Work out the finished part from the listing and answer in its coordinate system (mm). A direction names the side the tool comes from. Round coordinates to 2 decimals unless told otherwise and drop trailing zeros. Write each loop counter-clockwise with the first axis right and the second up, starting at its lowest first coordinate (ties: lowest second). Pieces come first, ordered by that corner, then holes.
1. A tool of negligible diameter and unlimited length cuts with its end or side. For faces 1 (the face through (103.216, 2.549, -5.514)), 2 (the face through (73.4, 1.6, -0.2)), 3 (the face through (15.24, 1.57, -18.86)), from which of +Z, -Z, +X, -X, +Y, -Y can it reach the whole face along a straight path? Write none if from no direction.
2. Find section B-B (y = 1.2). Count the separate pieces of the cut face and the enclosed holes in it, and give its area (3 significant figures).
3. Straight lines are drawn through the part: probe 1 along X at (y, z) = (0.65, -9.5); probe 2 along Z at (x, y) = (6.35, 1.8); probe 3 along X at (y, z) = (1.2, -10). For each, find the intervals that lie inside material, in ascending order.
4. Determine the mould class of faces 4 (the face through (56, 3.175, -10)), 5 (the face through (82.204, 2.549, -13.536)), 6 (the face through (0, 2, -10)) for opening direction X: pulls with the +X half, pulls with the -X half, needs draft (parallel to the pull), parting line crosses it, or undercut.
5. Find section C-C (x = 28). Write down the section's boundary in (y, z) (3 decimals), and give its area (3 significant figures).
6. Flat-ended cylindrical pins translate along their axes: pin 1 Ø2.5 at (x, z) = (92.71, -9.525) entering from -Y; pin 2 Ø6.5 at (x, z) = (88, -11) entering from +Y (3 decimals); pin 3 Ø1 at (y, z) = (1.5, -16) entering from +X; pin 4 Ø1.5 at (y, z) = (0.5, -3) entering from -X. Find the tip coordinate at first contact, or state that the pin passes through.
```python
from build123d import *

# Parameters (mm, degrees)
BOSS_EXTRUDE1_DEPTH          = 3.175
CUT_EXTRUDE2_DEPTH           = 1.27
F_1_8_0_125_DIAMETER_HOLE1_D = 3.175
CUT_EXTRUDE3_DEPTH           = 116.920115273
FILLET1_R                    = 15
F_1_8_0_125_DIAMETER_HOLE2_D = 3.175


with BuildPart() as part:
    # Sketch1 → Boss-Extrude1 (new body)
    with BuildSketch(Plane(origin=(0, 0, 0), x_dir=(1, 0, 0), z_dir=(0, 1, 0))):
        with BuildLine():
            Line((6.35, 0), (107.95, 0))
            ThreePointArc((107.95, 0), (112.440128061, 1.859871939), (114.3, 6.35))
            Line((114.3, 6.35), (114.3, 12.7))
            ThreePointArc((114.3, 12.7), (112.440128061, 17.190128061), (107.95, 19.05))
            Line((107.95, 19.05), (6.35, 19.05))
            ThreePointArc((6.35, 19.05), (1.859871939, 17.190128061), (0, 12.7))
            Line((0, 12.7), (0, 6.35))
            ThreePointArc((0, 6.35), (1.859871939, 1.859871939), (6.35, 0))
        make_face()
    extrude(amount=BOSS_EXTRUDE1_DEPTH)

    # Sketch4 → Cut-Extrude2 (cut)
    with BuildSketch(Plane(origin=(0, 3.175, 0), x_dir=(1, 0, 0), z_dir=(0, 1, 0))):
        with BuildLine():
            Line((109.744274308, 12.384881715), (96.868569632, 14.655215845))
            ThreePointArc((96.868569632, 14.655215845), (92.71, 16.129), (88.551430368, 14.655215845))
            Line((88.551430368, 14.655215845), (75.675725692, 12.384881715))
            ThreePointArc((75.675725692, 12.384881715), (73.276, 9.525), (75.675725692, 6.665118285))
            Line((75.675725692, 6.665118285), (88.551430368, 4.394784155))
            ThreePointArc((88.551430368, 4.394784155), (92.71, 2.921), (96.868569632, 4.394784155))
            Line((96.868569632, 4.394784155), (109.744274308, 6.665118285))
            ThreePointArc((109.744274308, 6.665118285), (112.144, 9.525), (109.744274308, 12.384881715))
        make_face()
    extrude(amount=-CUT_EXTRUDE2_DEPTH, mode=Mode.SUBTRACT)

    # 1/8 (0.125) Diameter Hole1 (through all)
    with Locations(Plane(origin=(0, 3.175, 0), x_dir=(1, 0, 0), z_dir=(0, 1, 0))):
        with Locations((6.35, 9.525)):
            Hole(F_1_8_0_125_DIAMETER_HOLE1_D / 2)

    # Sketch7 → Cut-Extrude3 (cut, through all)
    with BuildSketch(Plane(origin=(0, 3.175, 0), x_dir=(1, 0, 0), z_dir=(0, 1, 0))):
        with BuildLine():
            Line((15.415253533, 19.05), (73.276, 19.05))
            ThreePointArc((73.276, 19.05), (44.345626766, 13.880082039), (15.415253533, 19.05))
        make_face()
        with BuildLine():
            Line((73.276, 0), (15.415253533, 0))
            ThreePointArc((15.415253533, 0), (44.345626766, 5.169917961), (73.276, 0))
        make_face()
    extrude(amount=-CUT_EXTRUDE3_DEPTH, mode=Mode.SUBTRACT)

    # Fillet1
    fillet1_edges = [part.edges().sort_by_distance(p)[0] for p in [
        (73.276, 1.5875, -19.05),
        (15.415253533, 1.5875, -19.05),
        (15.415253533, 1.5875, 0),
        (73.276, 1.5875, 0),
    ]]
    fillet(fillet1_edges, radius=FILLET1_R)

    # 1/8 (0.125) Diameter Hole2 (through all)
    with Locations(Plane(origin=(0, 3.175, 0), x_dir=(1, 0, 0), z_dir=(0, 1, 0))):
        with Locations((92.71, 9.525)):
            Hole(F_1_8_0_125_DIAMETER_HOLE2_D / 2)


solid = part.part
```
Worked answers:
1. face 1: +Y
1. face 2: +Z, +Y, -Y
1. face 3: -Z, +Y, -Y
2. separate pieces: 1
2. enclosed holes: 2
2. area: 1,720 mm2
3. probe 1: x = 0 to 4.76, 7.94 to 91.12, 94.3 to 114.3
3. probe 2: z = -19.05 to -11.11, -7.94 to 0
3. probe 3: x = 0 to 4.84, 7.86 to 91.2, 94.22 to 114.3
4. face 4: needs draft
4. face 5: undercut
4. face 6: pulls with the -X half
5. outline: (0, -15.495) - (3.175, -15.495) - (3.175, -3.555) - (0, -3.555) - close
5. area: 37.9 mm2
6. pin 1: passes through
6. pin 2: stops at y = 1.905
6. pin 3: stops at x = 113.65
6. pin 4: stops at x = 0.56
